Here's how the part is built. I have some questions about the finished solid (model axes, mm). A direction names the side the tool comes from. Round coordinates to 2 decimals unless told otherwise and drop trailing zeros. Loops run counter-clockwise (first coordinate to the right, second up) from the corner with the lowest first, then second, coordinate; pieces in that order, holes last. Notation, with made-up numbers: M -9,65 L -3,65 A25 ccw -3,94 Z; hole C 39.25,82.25 d5. An arc over 180 degrees is marked long. One line per question, with ' | ' between items. Start each with the question number.
```python
from build123d import *

# Parameters (mm, degrees)
SKETCH1_R           = 15.55
SKETCH1_R_2         = 4.05
BOSS_EXTRUDE1_DEPTH = 4
CIRPATTERN1_COUNT   = 3


with BuildPart() as part:
    # Sketch1 → Boss-Extrude1 (new, symmetric)
    with BuildSketch(Plane(origin=(0, 0, 0), x_dir=(1, 0, 0), z_dir=(0, 1, 0))):
        with Locations(Location((0, 0, 0), (0, 0, 270))):
            Circle(SKETCH1_R)
        with Locations(Location((0, 0, 0), (0, 0, 270))):
            Circle(SKETCH1_R_2, mode=Mode.SUBTRACT)
    extrude(amount=BOSS_EXTRUDE1_DEPTH, both=True)

    # Sketch3 → Cut-Revolve1 (revolve, cut)
    with BuildSketch(Plane(origin=(0, 0, 0), x_dir=(1, 0, 0), z_dir=(0, 1, 0)), mode=Mode.PRIVATE) as cut_revolve1_sk:
        Polygon((15.55, 0), (15.55, 2.8), (12.05, 2.8), (12.05, 1.55), (8.55, 1.55), (8.55, 2.45), (1.114592602, 2.45), (1.114592602, 0), align=None)
    cut_revolve1 = revolve(cut_revolve1_sk.sketch.rotate(Axis((0, 0, 0), (1, 0, 0)), 180), axis=Axis((0, 0, 0), (1, 0, 0)), mode=Mode.SUBTRACT)

    # CirPattern1: Cut-Revolve1 ×3 about axis
    cirpattern1_axis = Axis((0, 0, 0), (0, 1, 0))
    for i in range(1, CIRPATTERN1_COUNT):
        add(cut_revolve1.rotate(cirpattern1_axis, i * 360 / CIRPATTERN1_COUNT), mode=Mode.SUBTRACT)


solid = part.part
```
1) Imagine slicing it at C-C (x = 13). Write out the boundary of the cut face in (y, z).
2) Imagine slicing it at A-A (z = 0). Write out the boundary of the cut face in (x, y).
3) For faces 4 (the face through (-4.8, 1.6, 7.1)), 5 (the face through (-3.954, -0.056, -0.878)), 6 (the face through (12.05, 1.21, 1.21)), which set-ups out of +Z, -Z, +X, -X, +Y, -Y let a thin tool reach every point of the face, with its end or its side?
4) I'm going to push flat-ended pins straight in: pin 1 Ø3 at (y, z) = (0, -0.5) entering from +X; pin 2 Ø4 at (x, y) = (10, -2.5) entering from -Z; pin 3 Ø3 at (x, y) = (12, 3) entering from -Z. Where does each tip first touch, or does it pass through?
5) Please list where these lines run through material, in increasing order: L1, parallel to Y at x = 11.3, z = 0; L2, parallel to X at y = 3.5, z = 0; L3, parallel to X at y = -1.75, z = 0. Write a range as from..to.
6) Imagine slicing it at B-B (y = 3.25). Write out the boundary of the cut face in (x, z), then the cut area to 3 significant figures.
7) Imagine slicing it at D-D (y = 1). State how many separate pieces and enclosed holes the cut face has, then the cut area to 3 significant figures.
8) We'd pull the mould along Z, two halves only. Please class faces 1 (the face through (-4.15, -1.05, 9.47)), 2 (the face through (-13.796, 0.056, 7.175)), 3 (the face through (-3, 4, 3)): pulls with the +Z half, pulls with the -Z half, needs draft (parallel to the pull), parting line crosses it, or undercut.
Results are:
1) outline: M -4,-8.53 L 4,-8.53 L 4,8.53 L -4,8.53 Z; hole C 0,0 d5.6
2) outline: M -15.55,-4 L -4.05,-4 L -4.05,4 L -15.55,4 Z; M 4.05,-4 L 15.55,-4 L 15.55,-2.8 L 12.05,-2.8 L 12.05,-1.55 L 8.55,-1.55 L 8.55,-2.45 L 4.05,-2.45 Z; M 4.05,2.45 L 8.55,2.45 L 8.55,1.55 L 12.05,1.55 L 12.05,2.8 L 15.55,2.8 L 15.55,4 L 4.05,4 Z
3) face 4: none | face 5: +Y, -Y | face 6: +X
4) pin 1: x = 12.05 | pin 2: z = -13.33 | pin 3: z = -11.47
5) L1: -4..-1.55, 1.55..4 | L2: -15.55..-4.05, 4.05..15.55 | L3: -15.55..-4.05, 8.55..12.05
6) outline: C 0,0 d31.1; hole C 0,0 d8.1 | area: 708 mm²
7) separate pieces: 3 | enclosed holes: 0 | area: 566 mm²
8) face 1: undercut | face 2: parting line crosses it | face 3: needs draft
